Design review of the part built by this model. Coordinates are the model's own, in mm. A direction names the side the tool comes from. Coordinates: 2 decimals unless noted, no trailing zeros. Loops run counter-clockwise (first coordinate to the right, second up) from the corner with the lowest first, then second, coordinate; pieces in that order, holes last. Notation, with made-up numbers: M 82,37 L 122,37 A20 cw 122,75 Z; hole C 1,34.5 d1. An arc over 180 degrees is marked long. Answer as a JSON object with one key per item and string values. Group by question number.
1. Insertion check: pin 1 (2 mm diameter, centred on x = -1.5, y = 2, fed in from +Z); pin 2 (8 mm diameter, centred on x = -4.5, z = 9.5, fed in from -Y); pin 3 (3 mm diameter, centred on x = 9.525, z = 0, fed in from +Y) (3 decimals); pin 4 (2 mm diameter, centred on y = 3.5, z = -9, fed in from +X). Each pin has a flat end and moves straight along its axis. Give the tip position at first contact, or say it passes through.
2. To check wall thickness, follow probe 1 along X at (y, z) = (8, 0); probe 2 along Y at (x, z) = (2.25, -5.25) (3 decimals); probe 3 along Z at (x, y) = (-5.75, 6). State the ranges of each line that lie inside material, in increasing order.
3. Consider section A-A (x = 0). State the section outline as (y, z) points (3 decimals).
4. Consider section C-C (y = 5.5). State the section outline as (x, z) points, then the cut area to 3 significant figures.
5. Draft analysis for pull direction Z (two halves, no side actions). For faces 3 (the cylindrical face through (-12.646, 6.306, -2.808)), 4 (the flat face through (13, 3.175, -2)), 5 (the flat face through (-5, 6.985, 8)), state which applies: +Z half, -Z half, draft (parallel to the pull), parting line (faces both ways), or undercut.
6. Machinability: for faces 1 (the flat face through (3, 9.525, 6)), 2 (the flat face through (-5, 6.985, -8)), which of the approach directions +Z, -Z, +X, -X, +Y, -Y give a long, thin tool a straight path to every point of the face, cutting with its end or side? Answer none if there is none.
7. Consider section D-D (y = 4). State the section outline as (x, z) points, then the cut area to 3 significant figures.
from build123d import *

# Parameters (mm, degrees)
SKETCH1_R           = 13.335
BOSS_EXTRUDE1_DEPTH = 3.175
SKETCH2_R           = 12.954
BOSS_EXTRUDE2_DEPTH = 6.35
SKETCH3_R           = 6.35
CUT_EXTRUDE2_DEPTH  = 5.08
SKETCH4_R           = 1.5875
CUT_EXTRUDE3_DEPTH  = 2.54
CIRPATTERN1_COUNT   = 3
FILLET1_R           = 2.54


with BuildPart() as part:
    # Sketch1 → Boss-Extrude1 (new body)
    with BuildSketch(Plane(origin=(0, 0, 0), x_dir=(1, 0, 0), z_dir=(0, 1, 0))):
        with Locations(Location((0, 0, 0), (0, 0, 270))):
            Circle(SKETCH1_R)
    extrude(amount=BOSS_EXTRUDE1_DEPTH)

    # Sketch2 → Boss-Extrude2 (add)
    with BuildSketch(Plane(origin=(0, 3.175, 0), x_dir=(1, 0, 0), z_dir=(0, 1, 0))):
        with Locations(Location((0, 0, 0), (0, 0, 270))):
            Circle(SKETCH2_R)
    extrude(amount=BOSS_EXTRUDE2_DEPTH)

    # Sketch3 → Cut-Extrude2 (cut)
    with BuildSketch(Plane(origin=(0, 9.525, 0), x_dir=(1, 0, 0), z_dir=(0, 1, 0))):
        with Locations(Location((0, 0, 0), (0, 0, 270))):
            Circle(SKETCH3_R)
    extrude(amount=-CUT_EXTRUDE2_DEPTH, mode=Mode.SUBTRACT)

    # Sketch4 → Cut-Extrude3 (cut)
    with BuildSketch(Plane(origin=(0, 9.525, 0), x_dir=(1, 0, 0), z_dir=(0, 1, 0))):
        with Locations(Location((9.525, 0, 0), (0, 0, 270))):
            Circle(SKETCH4_R)
    cut_extrude3 = extrude(amount=-CUT_EXTRUDE3_DEPTH, mode=Mode.SUBTRACT)

    # CirPattern1: Cut-Extrude3 ×3 about axis
    cirpattern1_axis = Axis((0, 0, 0), (0, 1, 0))
    for i in range(1, CIRPATTERN1_COUNT):
        add(cut_extrude3.rotate(cirpattern1_axis, i * 360 / CIRPATTERN1_COUNT), mode=Mode.SUBTRACT)

    # Fillet1
    fillet1_edges = [part.edges().sort_by_distance(p)[0] for p in [
        (0, 0, -13.335),
    ]]
    fillet(fillet1_edges, radius=FILLET1_R)


solid = part.part
Findings below:
{
 "1": {"pin 1": "stops at z = 13.32", "pin 2": "stops at y = 0", "pin 3": "stops at y = 6.985", "pin 4": "stops at x = 10.63"},
 "2": {"probe 1": "x = -12.95 to -6.35, 6.35 to 7.94, 11.11 to 12.95", "probe 2": "y = 0 to 4.445", "probe 3": "z = -11.61 to -2.69, 2.69 to 11.61"},
 "3": {"outline": "M 0,-10.795 A2.54 ccw 2.54,-13.335 L 3.175,-13.335 L 3.175,-12.954 L 9.525,-12.954 L 9.525,-6.35 L 4.445,-6.35 L 4.445,6.35 L 9.525,6.35 L 9.525,12.954 L 3.175,12.954 L 3.175,13.335 L 2.54,13.335 A2.54 ccw 0,10.795 Z"},
 "4": {"outline": "C 0,0 d25.91; hole C 0,0 d12.7", "area": "401 mm^2"},
 "5": {"face 3": "parting line", "face 4": "draft", "face 5": "undercut"},
 "6": {"face 1": "+Z, -Z, +X, -X, +Y", "face 2": "+Y"},
 "7": {"outline": "C 0,0 d25.91", "area": "527 mm^2"}
}
